The figure shows three views and two pictorial views of one solid part (mm, origin at its lowest corner). Answer the questions. Give positions to 0.01 mm unless a question says otherwise; leave off trailing zeros. Loops run counter-clockwise (first coordinate to the right, second up) from the corner with the lowest first, then second, coordinate; pieces in that order, holes last.
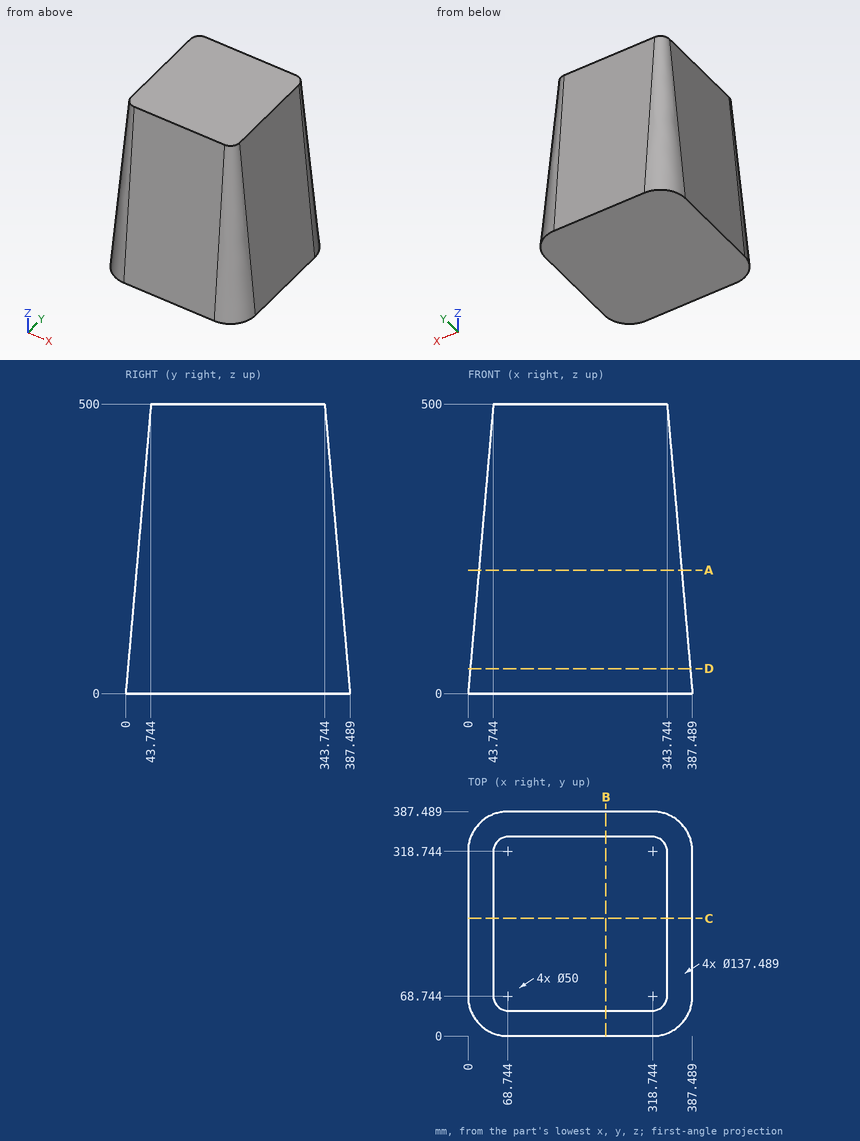
Q1. Section D-D on z = 43 is taken. Give the vertices of the cut face in (x, y) (1 decimal).
Q2. Given pin 1 (1 mm diameter, centred on y = 74, z = 431, fed in from +X) (1 decimal); pin 2 (12 mm diameter, centred on x = 174, z = 67, fed in from +Y); pin 3 (3 mm diameter, centred on y = 125, z = 212, fed in from -X), each flat-ended and moving along its own axis, determine where each tip first touches the part or whether it passes through.
Q3. Consider line 1 along X through (y, z) = (244.5, 219.5) (1 decimal); line 2 along X through (y, z) = (65, 196.5); line 3 along Y through (x, z) = (262.5, 46) (1 decimal). Determine where each line is inside the solid, lowest interval first.
Q4. Section B-B on x = 238 is taken. Give the vertices of the cut face in (y, z) (1 decimal).
Q5. Section A-A on z = 213 is taken. Give the vertices of the cut face in (x, y) (1 decimal), plus the area to 3 significant figures.
Check result:
1. outline: (3.8, 68.7) arc R65 ccw to (68.7, 3.8) - (318.7, 3.8) arc R65 ccw to (383.7, 68.7) - (383.7, 318.7) arc R65 ccw to (318.7, 383.7) - (68.7, 383.7) arc R65 ccw to (3.8, 318.7) - close
2. pin 1: stops at x = 349.8
2. pin 2: stops at y = 382.15
2. pin 3: stops at x = 18.42
3. line 1: x = 19.2 to 368.3
3. line 2: x = 17.33 to 370.16
3. line 3: y = 4 to 383.5
4. outline: (0, 0) - (387.5, 0) - (343.7, 500) - (43.7, 500) - close
5. outline: (18.6, 68.7) arc R50.1 ccw to (68.7, 18.6) - (318.7, 18.6) arc R50.1 ccw to (368.9, 68.7) - (368.9, 318.7) arc R50.1 ccw to (318.7, 368.9) - (68.7, 368.9) arc R50.1 ccw to (18.6, 318.7) - close
5. area: 120,000 mm2
